Source: CAD feature listing. Evaluate the final solid. Frame: model axes, mm. Face numbers are marked on the shaded views. A direction names the side the tool comes from. Round coordinates to 2 decimals unless told otherwise and drop trailing zeros. Loops run counter-clockwise (first coordinate to the right, second up) from the corner with the lowest first, then second, coordinate; pieces in that order, holes last. Notation, with made-up numbers: M -23,-30 L 33,-30 A12 cw 33,-12 Z; hole C -34.5,9 d7. An arc over 180 degrees is marked long. One line per item, written item: value.
from build123d import *

# Parameters (mm, degrees)
SKETCH_W       = 42
SKETCH_H       = 42
PAD_DEPTH      = 4.65
PAD_DEPTH_BACK = 0.4
POCKET_DEPTH   = 4.651


with BuildPart() as part:
    # Sketch → Pad (new body, two sides)
    with BuildSketch(Plane.XY) as pad_sk:
        Rectangle(SKETCH_W, SKETCH_H)
    extrude(amount=PAD_DEPTH)
    extrude(pad_sk.sketch, amount=-PAD_DEPTH_BACK)

    # SubtractivePipe: sweep along a path in Sketch001
    with BuildLine(Plane.XY) as subtractivepipe_path:
        Line((-17, -21), (17, -21))
        ThreePointArc((17, -21), (19.828427, -19.828427), (21, -17))
        Line((21, -17), (21, 17))
        ThreePointArc((21, 17), (19.828427, 19.828427), (17, 21))
        Line((17, 21), (-17, 21))
        ThreePointArc((-17, 21), (-19.828427, 19.828427), (-21, 17))
        Line((-21, 17), (-21, -17))
        ThreePointArc((-21, -17), (-19.828427, -19.828427), (-17, -21))
    # Sketch002 → SubtractivePipe (sweep, cut)
    with BuildSketch(Plane.XZ):
        Polygon((21, 4.65), (18.85, 2.5), (18.85, 0.7), (18.15, 0), (18.15, 4.65), align=None)
    sweep(path=subtractivepipe_path.line, mode=Mode.SUBTRACT)

    # Sketch003 → Pocket (cut, through all)
    with BuildSketch(Plane.XY):
        with BuildLine():
            Line((18.15, -17), (18.15, 17))
            ThreePointArc((18.15, 17), (17.813173, 17.813173), (17, 18.15))
            Line((17, 18.15), (-17, 18.15))
            ThreePointArc((-17, 18.15), (-17.813173, 17.813173), (-18.15, 17))
            Line((-18.15, 17), (-18.15, -17))
            ThreePointArc((-18.15, -17), (-17.813173, -17.813173), (-17, -18.15))
            Line((-17, -18.15), (17, -18.15))
            ThreePointArc((17, -18.15), (17.813173, -17.813173), (18.15, -17))
        make_face()
    extrude(amount=POCKET_DEPTH, mode=Mode.SUBTRACT)


solid = part.part
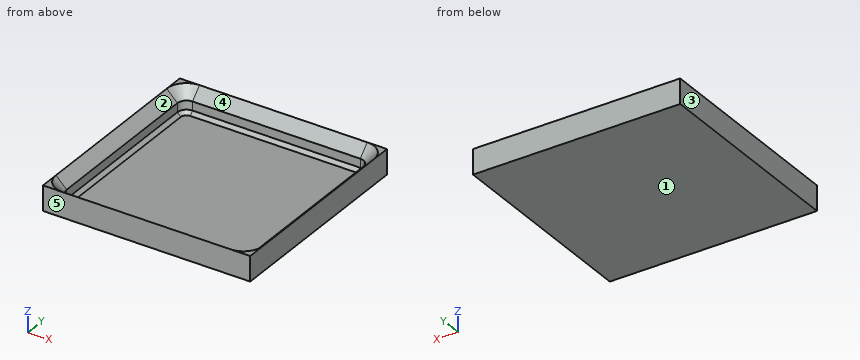
1. Pin query (flat end, axial travel): pin 1 (18 mm diameter, centred on x = 3, y = 7, fed in from +Z). Return the tip coordinate at first contact, or that it passes through.
Report:
pin 1: stops at z = 0
2. Section query D-D (z = 4.1). Return the cut outline in (x, y).
Report:
outline: M -21,-21 L 21,-21 L 21,21 L -21,21 Z; hole M -20.45,-17 A3.45 ccw -17,-20.45 L 17,-20.45 A3.45 ccw 20.45,-17 L 20.45,17 A3.45 ccw 17,20.45 L -17,20.45 A3.45 ccw -20.45,17 Z
3. Reachability of the marked faces 4 and 5 from +Z, -Z, +X, -X, +Y, -Y: full face, straight path, thin tool, end or side. Return the list, or none.
Report:
face 4: +Z
face 5: +Z, -Z, +X, -X, -Y
4. Section query A-A (z = 1.7). Return the cut outline in (x, y).
Report:
outline: M -21,-21 L 21,-21 L 21,21 L -21,21 Z; hole M -18.85,-17 A1.85 ccw -17,-18.85 L 17,-18.85 A1.85 ccw 18.85,-17 L 18.85,17 A1.85 ccw 17,18.85 L -17,18.85 A1.85 ccw -18.85,17 Z
5. Pull-direction query (X, two-part tool) for the marked faces 1, 2 and 3; classes: released by +X, released by -X, zero draft, split by the parting line, or undercut.
Report:
face 1: zero draft
face 2: undercut
face 3: released by -X
6. Section query B-B (x = 13). Return the cut outline in (y, z).
Report:
outline: M -21,-0.4 L 21,-0.4 L 21,4.65 L 18.85,2.5 L 18.85,0.7 L 18.15,0 L -18.15,0 L -18.85,0.7 L -18.85,2.5 L -21,4.65 Z
7. Ray query, line 1 (Y direction, x = 16, z = 1.7); line 2 (Z direction, x = -2, y = 16). Return the intervals inside material, ascending. Write a range as [from, to].
Report:
line 1: y = [-21, -18.85], [18.85, 21]
line 2: z = [-0.4, 0]
